Geometry check sheet. Reference: the model listing, model coordinates, mm. A direction names the side the tool comes from. Give positions to 0.01 mm unless a question says otherwise; leave off trailing zeros. Write each loop counter-clockwise with the first axis right and the second up, starting at its lowest first coordinate (ties: lowest second). Pieces come first, ordered by that corner, then holes. Notation, with made-up numbers: (10, -21) -> (33, -21) arc R21 ccw to (33, 1) -> close; hole circle Ø1 at (48, 67.5). An arc over 180 degrees is marked (long way). Write item = value, one per line. Start each with the question number.
1. Cross-section at C-C, the plane x = 16. Record the cut outline in (y, z), plus the area to 3 significant figures.
2. Cross-section at A-A, the plane z = 15.5. Record the cut outline in (x, y).
3. Set-up check for faces 5 (the flat face through (-12, 15, -21.5)), 6 (the cylindrical face through (4.979, 14.79, -29.545)): record each of +Z, -Z, +X, -X, +Y, -Y from which the full face is reachable in a straight line by a thin tool's end or side.
4. Mould release check, pull along X, two halves, no side actions. Record for faces 1 (the flat face through (-1.5, 15, -6)), 2 (the cylindrical face through (-11.83, 2.46, 21.48)), 3 (the cylindrical face through (26.1, 14.79, -29.21)), 4 (the flat face through (16, 15, 9)): pulls with the +X half, pulls with the -X half, needs draft (parallel to the pull), parting line crosses it, or undercut.
5. Thickness scan on line 1 along Z through (x, y) = (-11.5, 3.2); line 2 along Y through (x, z) = (-16.5, -20.5); line 3 along Z through (x, y) = (4, 28.25). Record the ranges inside material, lowest first.
6. Cross-section at B-B, the plane x = -11.5. State how many separate pieces and enclosed holes the cut face has, plus the area to 3 significant figures.
7. Depth check by flat-ended pin: P1, Ø6, axis at y = 18, z = -11, coming from the -X side; P2, Ø5.5, axis at x = -8.5, y = 12.5, coming from the +Z side. Enter the tip coordinate at first touch or a pass-through.
8. Cross-section at D-D, the plane x = 23.5. Record the cut outline in (y, z).
Autodesk Inventor part; units mm, degrees
ref_plane "YZ Plane" through (0, 0, 0) normal (1, 0, 0) x (0, 1, 0)
ref_plane "XZ Plane" through (0, 0, 0) normal (0, 1, 0) x (-1, 0, 0)
ref_plane "XY Plane" through (0, 0, 0) normal (0, 0, 1) x (1, 0, 0)
sketch "Sketch1" plane through (0, 0, 0) normal (0, 1, 0) x (-1, 0, 0)
  line L0 (-2, 0) -> (-30, 0)
  line L1 (-32, -2) -> (-32, -30)
  line L2 (-30, -32) -> (-2, -32)
  line L3 (0, -30) -> (0, -2)
  circle A0 centre (-16, -16) radius 10.5
  line L4 (1.5, -41) -> (-33.5, -41)
  line L5 (-33.5, -41) -> (-33.5, 9)
  line L6 (-33.5, 9) -> (1.5, 9)
  line L7 (1.5, 9) -> (1.5, -41)
  line L8 (1.5, -41) -> (-33.5, 9) construction
  line L9 (-33.5, -41) -> (1.5, 9) construction
  circle A1 centre (-16, -16) radius 16 construction
  line L10 (-2, -32) -> (0, -30)
  line L11 (0, -2) -> (-2, 0)
  line L12 (-30, 0) -> (-32, -2)
  line L13 (-30, -32) -> (-32, -30)
  line L14 (-16, -16) -> (0, 0) construction
  line L15 (-16, -16) -> (-32, 0) construction
  line L16 (-16, -16) -> (-32, -32) construction
  circle A2 centre (-27.3137, -27.3137) radius 2.25
  line L17 (-16, -16) -> (0, -32) construction
  circle A3 centre (-4.6863, -27.3137) radius 2.25
  circle A4 centre (-4.6863, -4.6863) radius 2.25
  circle A5 centre (-27.3137, -4.6863) radius 2.25
  line L18 (1.5, -41) -> (21.5, -41)
  line L19 (21.5, -41) -> (21.5, -21.5)
  line L20 (21.5, -21.5) -> (1.5, -21.5)
  line L21 (1.5, -21.5) -> (1.5, -41)
  point P0 (-33.5, -36)
  point P1 (1.5, -36)
  dimension "d0" = 32
  dimension "d1" = 32
  dimension "d2" = 21
  dimension "d3" = 16
  dimension "d4" = 16
  dimension "d5" = 35
  dimension "d6" = 50
  dimension "d10" = 32
  dimension "d15" = 2
  dimension "d16" = 2
  dimension "d17" = 2
  dimension "d18" = 2
  dimension "d19" = 2
  dimension "d20" = 2
  dimension "d21" = 2
  dimension "d22" = 2
  dimension "d56" = 4.5
  dimension "d57" = 4.5
  dimension "d58" = 4.5
  dimension "d59" = 4.5
  dimension "d63" = 20
  dimension "d64" = 19.5
extrude "Extrusion1" add sketch "Sketch1" along normal blind 30 contours L11 L3 L10 L2 L13 L1 L12 L0 | L4 L5 L6 L7
sketch "Sketch3" plane through (-1.5, 0, 9) normal (0, 0, 1) x (1, 0, 0)
  line L0 (35, 0) -> (35, 30)
  line L1 (0, 0) -> (35, 0)
  line L2 (35, 0) -> (35, 5)
  line L3 (35, 5) -> (0, 5)
  line L4 (0, 5) -> (0, 0)
  point P0 (1.5, 0)
  dimension "d27" = 5
extrude "Extrusion2" add sketch "Sketch3" along normal blind 20
sketch "Sketch4" plane through (-1.5, 0, -41) normal (-1, 0, 0) x (0, 0, 1)
  line L0 (0, 0) -> (0, 30)
  line L1 (50, 5) -> (70, 5)
  line L2 (0, 0) -> (70, 0)
  line L3 (70, 0) -> (70, 5)
  line L4 (70, 5) -> (0, 5)
  line L5 (0, 5) -> (0, 0)
  point P0 (41, 0)
extrude "Extrusion3" add sketch "Sketch4" along normal blind 20
sketch "Sketch5" plane through (-1.5, 30, 9) normal (0, 0, 1) x (1, 0, 0)
  line L0 (35, 0) -> (0, 0)
  line L1 (0, -25) -> (0, 0)
  line L2 (35, 0) -> (0, 0)
  line L3 (0, 0) -> (0, -5)
  line L4 (0, -5) -> (35, -5)
  line L5 (35, -5) -> (35, 0)
  point P0 (1.5, -30)
  dimension "d33" = 5
extrude "Extrusion4" add sketch "Sketch5" along normal blind 20
sketch "Sketch6" plane through (-1.5, 5, -41) normal (-1, 0, 0) x (0, 0, 1)
  line L0 (50, 20) -> (70, 20)
  line L1 (0, 0) -> (0, 25)
  line L2 (70, 20) -> (0, 20)
  line L3 (0, 20) -> (0, 25)
  line L4 (0, 25) -> (70, 25)
  line L5 (70, 25) -> (70, 20)
  point P0 (41, -5)
extrude "Extrusion5" add sketch "Sketch6" along normal blind 20
sketch "Sketch7" plane through (0, 0, 0) normal (0, -1, 0) x (1, 0, 0)
  circle A0 centre (-11.5, 19) radius 2.5
  circle A1 centre (6, 19) radius 2.5
  circle A2 centre (23.5, 19) radius 2.5
  circle A3 centre (-11.5, -6) radius 2.5
  line L0 (33.5, 29) -> (-21.5, 29) construction
  line L1 (33.5, -41) -> (33.5, 29) construction
  line L2 (-21.5, 29) -> (33.5, 29) construction
  line L3 (33.5, 29) -> (33.5, -41) construction
  line L4 (33.5, -41) -> (-21.5, -41) construction
  line L5 (-21.5, -41) -> (-21.5, 29) construction
  line L6 (-1.5, -41) -> (-21.5, -41) construction
  line L7 (-11.5, 19) -> (-21.5, 19) construction
  line L8 (-11.5, 19) -> (-11.5, 29) construction
  line L9 (-11.5, 19) -> (-11.5, -6) construction
  line L10 (-11.5, 19) -> (6, 19) construction
  line L11 (6, 19) -> (23.5, 19) construction
  line L12 (-21.5, -21.5) -> (-1.5, -21.5)
  line L13 (-1.5, -21.5) -> (-1.5, -41)
  point P0 (0, 0)
  dimension "d41" = 5
  dimension "d44" = 5
  dimension "d45" = 5
  dimension "d48" = 5
  dimension "d51" = 17.5
  dimension "d60" = 25
  dimension "d71" = 10
  dimension "d72" = 10
  dimension "d73" = 17.5
  dimension "d74" = 20
  dimension "d75" = 19.5
extrude "Extrusion6" cut sketch "Sketch7" against normal blind 30
extrude "Extrusion7" add sketch "Sketch1" along normal blind 25 contours L7 L20 L19 L18
sketch "Sketch9" plane through (33.5, 0, -41) normal (0, 0, -1) x (-1, 0, 0)
  line L0 (0, 0) -> (0, 5)
  line L1 (0, 0) -> (55, 0)
  line L2 (55, 0) -> (55, 30)
  line L3 (55, 30) -> (0, 30)
  line L4 (0, 30) -> (0, 0)
  point P0 (33.5, 0)
  dimension "d76" = 55
  dimension "d77" = 30
extrude "Extrusion8" cut sketch "Sketch9" against normal blind 5
fillet "Fillet3" radius 1 26 edges at (33.5, 0, -3.5) (33.5, 30, -3.5) (33.5, 15, 9) (33.5, 25, 19) (6, 25, 29) (33.5, 27.5, 29) (6, 30, 29) (-21.5, 27.5, 29) (-21.5, 25, 3.75) (-21.5, 30, -3.5) (-21.5, 15, -21.5) (-21.5, 5, 3.75) (-21.5, 2.5, 29) (6, 5, 29) (6, 0, 29) (-21.5, 0, -3.5) (33.5, 2.5, 29) (33.5, 15, -36) (6, 0, -36) (-21.5, 15, -36) (6, 30, -36) (-1.5, 15, 9) (-1.5, 15, -21.5) (-11.5, 25, -21.5) (-11.5, 5, -21.5) (33.5, 5, 19)
equation "\"d16\" = d15"
equation "\"d17\" = d15"
equation "\"d18\" = d17"
equation "\"d21\" = d15"
equation "\"d22\" = d21"
properties part number "bed_pulley_holder" material "Plastic, Opaque Black"
Answers:
q1.outline = (0, -35) arc R1 ccw to (1, -36) -> (29, -36) arc R1 ccw to (30, -35) -> (30, -26.5) -> (0, -26.5) -> close; (0, -5.5) -> (30, -5.5) -> (30, 28) arc R1 ccw to (29, 29) -> (26, 29) arc R1 ccw to (25, 28) -> (25, 9) -> (5, 9) -> (5, 28) arc R1 ccw to (4, 29) -> (1, 29) arc R1 ccw to (0, 28) -> close
q1.area = 919 mm^2
q2.outline = (-21.5, 1) arc R1 ccw to (-20.5, 0) -> (32.5, 0) arc R1 ccw to (33.5, 1) -> (33.5, 4) arc R1 ccw to (32.5, 5) -> (-20.5, 5) arc R1 ccw to (-21.5, 4) -> close; (-21.5, 26) arc R1 ccw to (-20.5, 25) -> (32.5, 25) arc R1 ccw to (33.5, 26) -> (33.5, 29) arc R1 ccw to (32.5, 30) -> (-20.5, 30) arc R1 ccw to (-21.5, 29) -> close
q3.face_5 = +Z, -X
q3.face_6 = +Y, -Y
q4.face_1 = pulls with the -X half
q4.face_2 = undercut
q4.face_3 = undercut
q4.face_4 = needs draft
q5.line_1 = -36 to -8.5, -3.5 to 16.5, 21.5 to 29
q5.line_2 = 0 to 5, 25 to 30
q5.line_3 = -36 to -29.46, -25.17 to -6.83, -2.54 to 17.5, 20.5 to 29
q6.separate_pieces = 5
q6.enclosed_holes = 0
q6.area = 839 mm^2
q7.P1 = -1.5
q7.P2 = -21.5
q8.outline = (0, -35) arc R1 ccw to (1, -36) -> (29, -36) arc R1 ccw to (30, -35) -> (30, -23.35) -> (0, -23.35) -> close; (0, -8.65) -> (30, -8.65) -> (30, 16.5) -> (25, 16.5) -> (25, 9) -> (5, 9) -> (5, 16.5) -> (0, 16.5) -> close; (0, 21.5) -> (5, 21.5) -> (5, 28) arc R1 ccw to (4, 29) -> (1, 29) arc R1 ccw to (0, 28) -> close; (25, 21.5) -> (30, 21.5) -> (30, 28) arc R1 ccw to (29, 29) -> (26, 29) arc R1 ccw to (25, 28) -> close
